Design review of the part built by this model. Coordinates are the model's own, in mm. A direction names the side the tool comes from. Coordinates: 2 decimals unless noted, no trailing zeros. Loops run counter-clockwise (first coordinate to the right, second up) from the corner with the lowest first, then second, coordinate; pieces in that order, holes last.
Q1. Add section C-C on y = 63.5. Give the boundary of the cut face in (x, z).
Q2. Add section B-B on z = 6.5. Give the boundary of the cut face in (x, y).
Q3. Draft analysis for pull direction Z (two halves, no side actions). For faces 1 (the face through (24.2, 1, 7)), 2 (the face through (-1, 2, 0)), 3 (the face through (-8, 79, 15.2)), state which applies: released by +Z, released by -Z, zero draft, split by the parting line, or undercut.
Q4. Add section A-A on x = 2. Give the boundary of the cut face in (y, z).
Q5. For P1, Ø10, axis at x = 13, y = -67, coming from the +Z side; P2, Ø1.1, axis at y = 79.5, z = 16.5, coming from the -X side; P3, Ø4, axis at x = 28.5, z = 4, coming from the -Y side; P4, Ø1.9, axis at x = -4, z = 17, coming from the -Y side, all flat-tipped, find the tip position at first contact; note any pin that passes through.
Q6. Add section D-D on x = 34.5. Give the boundary of the cut face in (y, z), and give its area (3 significant figures).
Q7. Wall thickness on probe 1 along Z at (x, y) = (19, -75); probe 2 along Z at (x, y) = (27.5, 76.5); probe 3 along X at (y, z) = (-16.5, 14.75): over which ranges is each line inside the solid? List them lowest first.
Q8. Machinability: for faces 4 (the face through (-9, -112.4, 2)), 5 (the face through (-8, -79, 15.2)), 6 (the face through (6, -87.1, 7)), 7 (the face through (-32, 2, 3)), 8 (the face through (6, 87.1, 7)), which of the approach directions +Z, -Z, +X, -X, +Y, -Y give a long, thin tool a straight path to every point of the face, cutting with its end or side? Answer none if there is none.
```python
from build123d import *

# Parameters (mm, degrees)
F0_W      = 78.6
F0_H      = 224.8
F1_DEPTH  = 3
F2_W      = 13.4
F2_H      = 14.6
F3_DEPTH  = 224.8
F5_W      = 35.1
F5_H      = 8.8
F6_DEPTH  = 174
F8_DEPTH  = 15.5
F12_DEPTH = 7.4
F15_DEPTH = 7.4


with BuildPart() as f1:
    # F0 (on Top) → F1 (new body)
    with BuildSketch(Plane.XY):
        Rectangle(F0_W, F0_H)
    extrude(amount=F1_DEPTH)

    # F2 (on face) → F3 (join, through all)
    with BuildSketch(Plane.XZ.offset(112.4)):
        with Locations((-17.6, 10.3)):
            Rectangle(F2_W, F2_H)
    extrude(amount=-F3_DEPTH)

    # F5 (on offset) → F6 (join)
    with BuildSketch(Plane.XZ.offset(86.9)):
        with Locations((6.65, 7.4)):
            Rectangle(F5_W, F5_H)
    extrude(amount=-F6_DEPTH)

    # F7 (on offset) → F8 (join)
    with BuildSketch(Plane.XZ.offset(86.9)):
        Polygon((-10.9, 17.6), (-10.9, 15.2), (-3.2, 15.2), (-0.6, 17.6), align=None)
    extrude(amount=-F8_DEPTH)

    # F9: F1 across plane


with BuildPart() as f1_1:
    add(f1.part)
    add(f1.part.mirror(Plane.XZ))

    # F11 (on offset) → F12 (cut)
    with BuildSketch(Plane.XZ.offset(85.2)):
        Polygon((-6.8416666667, 16.9), (-6.8416666667, 15.2), (-3.2, 15.2), (-2.4416666667, 15.9), (-3.7416666667, 15.9), (-3.7416666667, 16.9), align=None)
    extrude(amount=-F12_DEPTH, mode=Mode.SUBTRACT)

    # F14 (on offset) → F15 (cut)
    with BuildSketch(Plane.XZ.offset(-75.4)):
        Polygon((-6.8416666667, 16.9), (-6.8416666667, 15.2), (-3.2, 15.2), (-2.4416666667, 15.9), (-3.7416666667, 15.9), (-3.7416666667, 16.9), align=None)
    extrude(amount=-F15_DEPTH, mode=Mode.SUBTRACT)


solid = f1_1.part
```
Entries:
1. outline: (-39.3, 0) - (39.3, 0) - (39.3, 3) - (24.2, 3) - (24.2, 11.8) - (-10.9, 11.8) - (-10.9, 17.6) - (-24.3, 17.6) - (-24.3, 3) - (-39.3, 3) - close
2. outline: (-24.3, -112.4) - (-10.9, -112.4) - (-10.9, -87.1) - (24.2, -87.1) - (24.2, 87.1) - (-10.9, 87.1) - (-10.9, 112.4) - (-24.3, 112.4) - close
3. face 1: zero draft
3. face 2: released by -Z
3. face 3: undercut
4. outline: (-112.4, 0) - (112.4, 0) - (112.4, 3) - (87.1, 3) - (87.1, 11.8) - (-87.1, 11.8) - (-87.1, 3) - (-112.4, 3) - close
5. P1: stops at z = 11.8
5. P2: stops at x = -24.3
5. P3: stops at y = -112.4
5. P4: stops at y = -86.9
6. outline: (-112.4, 0) - (112.4, 0) - (112.4, 3) - (-112.4, 3) - close
6. area: 674 mm2
7. probe 1: z = 0 to 11.8
7. probe 2: z = 0 to 3
7. probe 3: x = -24.3 to -10.9
8. face 4: +Z, -Z, +X, -X, -Y
8. face 5: +X, +Y, -Y
8. face 6: +Z, +X, -Y
8. face 7: +Z, -X, +Y, -Y
8. face 8: +Z, +X, +Y
